from build123d import *

# Parameters (mm, degrees)
SKETCH2_R           = 4
BOSS_EXTRUDE1_DEPTH = 20
SKETCH3_W           = 25
SKETCH3_H           = 25
CUT_EXTRUDE1_DEPTH  = 107.529597523


with BuildPart() as part:
    # Sketch2 → Boss-Extrude1 (new, symmetric)
    with BuildSketch(Plane(origin=(0, 0, 0), x_dir=(1, 0, 0), z_dir=(0, 1, 0))):
        with BuildLine():
            Line((-30.805843601, 0), (-70, 0))
            ThreePointArc((-70, 0), (-73.109650812, 1.084636437), (-74.870165393, 3.867971269))
            Line((-74.870165393, 3.867971269), (-85.606821951, 50.05875403))
            ThreePointArc((-85.606821951, 50.05875403), (-83.158089611, 57.823709992), (-75.174557322, 59.421847456))
            Line((-75.174557322, 59.421847456), (49.836959924, 15.71990466))
            ThreePointArc((49.836959924, 15.71990466), (51.797432477, 14.458972094), (52.973218852, 12.446279875))
            Line((52.973218852, 12.446279875), (54.786258928, 6.446279875))
            ThreePointArc((54.786258928, 6.446279875), (54.01443641, 2.019345657), (50, 0))
            Line((50, 0), (30.805843601, 0))
            ThreePointArc((30.805843601, 0), (0, 13), (-30.805843601, 0))
        make_face()
        with Locations(Location((-77.814557322, 51.87, 0), (0, 0, 270))):
            Circle(SKETCH2_R, mode=Mode.SUBTRACT)
        with Locations(Location((-73.36, 27, 0), (0, 0, 270))):
            Circle(SKETCH2_R, mode=Mode.SUBTRACT)
    extrude(amount=BOSS_EXTRUDE1_DEPTH, both=True)

    # Sketch3 → Cut-Extrude1 (cut, through all)
    with BuildSketch(Plane.XY):
        with Locations((-73.314557322, 0)):
            Rectangle(SKETCH3_W, SKETCH3_H)
    extrude(amount=-CUT_EXTRUDE1_DEPTH, mode=Mode.SUBTRACT)


solid = part.part
Check sheet for the modelled part. Datum: model origin and axes. Units: mm. A direction names the side the tool comes from. Round coordinates to 2 decimals unless told otherwise and drop trailing zeros. Order: outer loops, then holes, each group sorted by start corner. A loop starts at its lowest first (then second) coordinate and runs counter-clockwise, first axis right, second up.
(1) Cross-section at A-A, the plane z = -25.5. Enter the section's corners in (x, y).
(2) Scan lines: probe 1 along Y at (x, z) = (-74.5, -36.5); probe 2 along X at (y, z) = (5.5, -3.5); probe 3 along X at (y, z) = (-16.5, -5). Record each from-to range of solid material in increasing order.
(3) Cross-section at C-C, the plane y = 1.5. Enter the section's corners in (x, z).
(4) Cross-section at D-D, the plane z = -34. Enter the section's corners in (x, y), and give its area (3 significant figures).
(5) Draft check along Z on faces 1 (the flat face through (-50, 0, 0)), 2 (the cylindrical face through (-81.36, -16.3, -50.02)), 3 (the cylindrical face through (-81.36, 16.2, -50.02)), 4 (the flat face through (-30, 20, -24)). Enter one of: pulls with the +Z half, pulls with the -Z half, needs draft (parallel to the pull), parting line crosses it, or undercut.
(6) Access from +Z, -Z, +X, -X, +Y, -Y to the whole of each face (thin tool, end or side, straight path). Record for faces 5 (the flat face through (-80.163, 16.303, -26.64)), 6 (the flat face through (-68, 12.5, -30)).
(7) Cross-section at B-B, the plane y = -14. Enter the section's corners in (x, z).
(8) Go/stop test with flat-tipped pins: P1, Ø4, axis at y = 15, z = -23.5, coming from the -X side; P2, Ø1, axis at x = -25, y = -7, coming from the +Z side; P3, Ø12.5, axis at y = 1.5, z = -15, coming from the -X side. Record where each tip stops, or that it passes through.
Check sheet entries:
1. outline: (-79.9, -20) - (-77.07, -20) - (-77.07, -12.5) - (-79.9, -12.5) - close; (-79.9, 12.5) - (-77.07, 12.5) - (-77.07, 20) - (-79.9, 20) - close; (-69.65, -20) - (21.86, -20) - (21.86, 20) - (-69.65, 20) - (-69.65, 12.5) - (-60.81, 12.5) - (-60.81, -12.5) - (-69.65, -12.5) - close
2. probe 1: y = -20 to -12.5, 12.5 to 20
2. probe 2: x = -60.81 to -26.96, 26.96 to 54.77
2. probe 3: x = -75.13 to -24.98, 24.98 to 55
3. outline: (-60.81, -54.4) - (49.84, -15.72) arc R5 ccw to (52.97, -12.45) - (54.79, -6.45) arc R5 ccw to (50, 0) - (30.81, 0) arc R43 cw to (-30.81, 0) - (-60.81, 0) - close
4. outline: (-81.87, -20) - (-2.45, -20) - (-2.45, 20) - (-81.87, 20) - (-81.87, 12.5) - (-60.81, 12.5) - (-60.81, -12.5) - (-81.87, -12.5) - close
4. area: 2,650 mm2
5. face 1: pulls with the +Z half
5. face 2: undercut
5. face 3: undercut
5. face 4: needs draft
6. face 5: +Z, -X, +Y, -Y
6. face 6: +Z, -Z, -X
7. outline: (-85.61, -50.06) arc R8 ccw to (-75.17, -59.42) - (49.84, -15.72) arc R5 ccw to (52.97, -12.45) - (54.79, -6.45) arc R5 ccw to (50, 0) - (30.81, 0) arc R43 cw to (-30.81, 0) - (-70, 0) arc R5 ccw to (-74.87, -3.87) - close; hole circle Ø8 at (-77.81, -51.87); hole circle Ø8 at (-73.36, -27)
8. P1: stops at x = -79.9
8. P2: stops at z = -4.62
8. P3: stops at x = -60.81
